Check sheet for the drawn part. Datum: minimum x, y, z corner. Units: mm. Give positions to 0.01 mm unless a question says otherwise; leave off trailing zeros. Order: outer loops, then holes, each group sorted by start corner. A loop starts at its lowest first (then second) coordinate and runs counter-clockwise, first axis right, second up. Notation, with made-up numbers: (-34.75, 29) - (-6.75, 29) arc R21 ccw to (-6.75, 41) - close; hole circle Ø7 at (36, 54.5). An arc over 180 degrees is marked (long way). Answer as a JSON object with one key per item and string values. Group by question number.
(1) Depth check by flat-ended pin: pin 1 Ø1 at (x, z) = (27.5, 25.5) entering from -Y. Enter the tip coordinate at first touch or a pass-through.
(2) Section check B-B (z = 12). Record the boundary of the cut face in (x, y), then the cut area to 3 significant figures.
(3) Section check A-A (x = 64). Record the boundary of the cut face in (y, z).
(4) Section check D-D (x = 9.5). Record the boundary of the cut face in (y, z).
(5) Thickness scan on line 1 (X direction, y = 1.6, z = 12); line 2 (X direction, y = 0.3, z = 10.5); line 3 (Z direction, x = 64, y = 1). Record the ranges inside material, lowest first.
(6) Section check C-C (y = 0.7). Record the boundary of the cut face in (x, z), then the cut area to 3 significant figures.
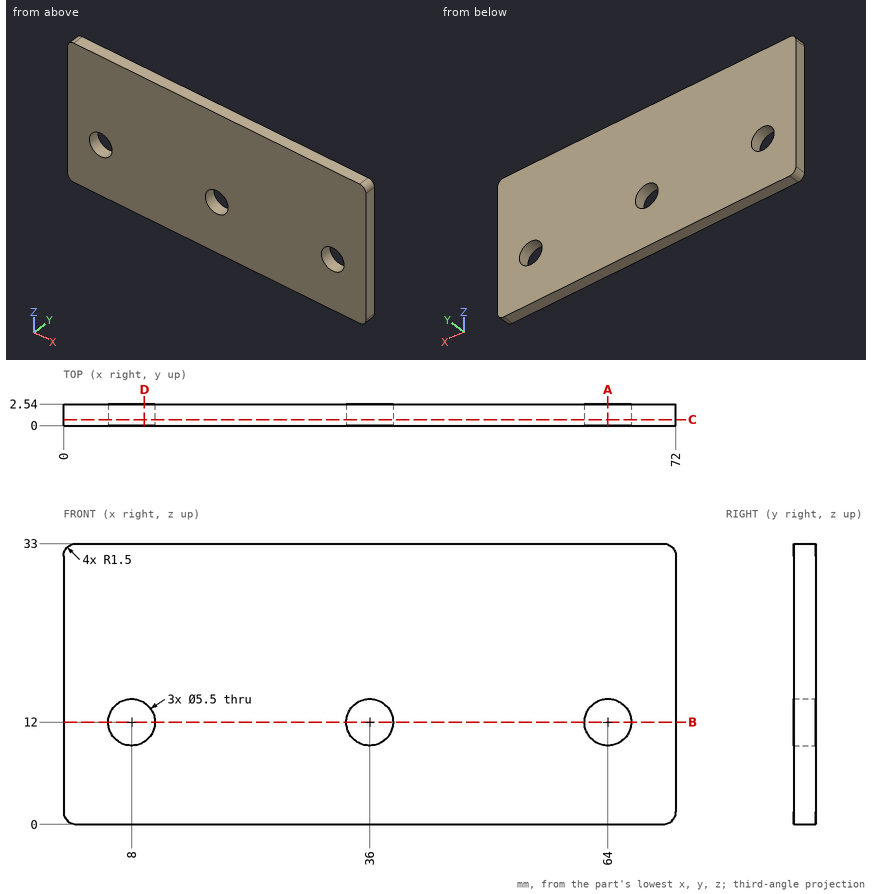
Solutions:
{
 "1": {"pin 1": "stops at y = 0"},
 "2": {"outline": "(0, 0) - (5.25, 0) - (5.25, 2.54) - (0, 2.54) - close; (10.75, 0) - (33.25, 0) - (33.25, 2.54) - (10.75, 2.54) - close; (38.75, 0) - (61.25, 0) - (61.25, 2.54) - (38.75, 2.54) - close; (66.75, 0) - (72, 0) - (72, 2.54) - (66.75, 2.54) - close", "area": "141 mm2"},
 "3": {"outline": "(0, 0) - (2.54, 0) - (2.54, 9.25) - (0, 9.25) - close; (0, 14.75) - (2.54, 14.75) - (2.54, 33) - (0, 33) - close"},
 "4": {"outline": "(0, 0) - (2.54, 0) - (2.54, 9.7) - (0, 9.7) - close; (0, 14.3) - (2.54, 14.3) - (2.54, 33) - (0, 33) - close"},
 "5": {"line 1": "x = 0 to 5.25, 10.75 to 33.25, 38.75 to 61.25, 66.75 to 72", "line 2": "x = 0 to 5.7, 10.3 to 33.7, 38.3 to 61.7, 66.3 to 72", "line 3": "z = 0 to 9.25, 14.75 to 33"},
 "6": {"outline": "(0, 1.5) arc R1.5 ccw to (1.5, 0) - (70.5, 0) arc R1.5 ccw to (72, 1.5) - (72, 31.5) arc R1.5 ccw to (70.5, 33) - (1.5, 33) arc R1.5 ccw to (0, 31.5) - close; hole circle Ø5.5 at (8, 12); hole circle Ø5.5 at (36, 12); hole circle Ø5.5 at (64, 12)", "area": "2,300 mm2"}
}
